Build history of the part. All positions in model axes, mm. Coordinates: 2 decimals unless noted, no trailing zeros. Write each loop counter-clockwise with the first axis right and the second up, starting at its lowest first coordinate (ties: lowest second). Pieces come first, ordered by that corner, then holes. Notation, with made-up numbers: (72, 12.25) -> (95, 12.25) arc R30 cw to (95, 39.25) -> close; hole circle Ø8 at (6.25, -29). An arc over 180 degrees is marked (long way). Write each question's results on one line, items separated by ' | '. Start each with the question number.
Q1. Drill centre lines: line 1 (Z direction, x = 3.25, y = -1.45); line 2 (Y direction, x = -0.5, z = 1.8); line 3 (X direction, y = 0.5, z = 1.8). Where is each one in solid material? Low to high.
Q2. Saw through at B-B on z = 0.75. Give the cut face in (x, y) (1 decimal), and give its area (3 significant figures).
Q3. Saw through at C-C on z = 1.45. Give the cut face in (x, y), and give its area (3 significant figures).
Q4. Saw through at A-A on x = -1. Give the cut face in (y, z) (1 decimal), and give its area (3 significant figures).
Q5. Saw through at D-D on y = -1.65. Give the cut face in (x, z).
from build123d import *

# Parameters (mm, degrees)
F0_W     = 9.906
F0_H     = 4.191
F1_DEPTH = 1.27
F3_DEPTH = 0.635
F4_R     = 0.3175
F5_DEPTH = 25.4


with BuildPart() as f1:
    # F0 (on Top) → F1 (new body)
    with BuildSketch(Plane.XY):
        Rectangle(F0_W, F0_H)
    extrude(amount=F1_DEPTH)

    # F2 (on face) → F3 (join)
    with BuildSketch(Plane.XY.offset(1.27)):
        with BuildLine():
            ThreePointArc((3.81, 0), (3.438026, 0.898026), (2.54, 1.27))
            Line((2.54, 1.27), (-2.54, 1.27))
            ThreePointArc((-2.54, 1.27), (-3.438026, 0.898026), (-3.81, 0))
            ThreePointArc((-3.81, 0), (-3.438026, -0.898026), (-2.54, -1.27))
            Line((-2.54, -1.27), (2.54, -1.27))
            ThreePointArc((2.54, -1.27), (3.438026, -0.898026), (3.81, 0))
        make_face()
    extrude(amount=F3_DEPTH)

    # F4 (on face) → F5 (cut)
    with BuildSketch(Plane.XY.offset(1.27)):
        with Locations((4.422641, 0)):
            Circle(F4_R)
        with Locations((-4.389373, 0)):
            Circle(F4_R)
    extrude(amount=-F5_DEPTH, mode=Mode.SUBTRACT)


solid = f1.part
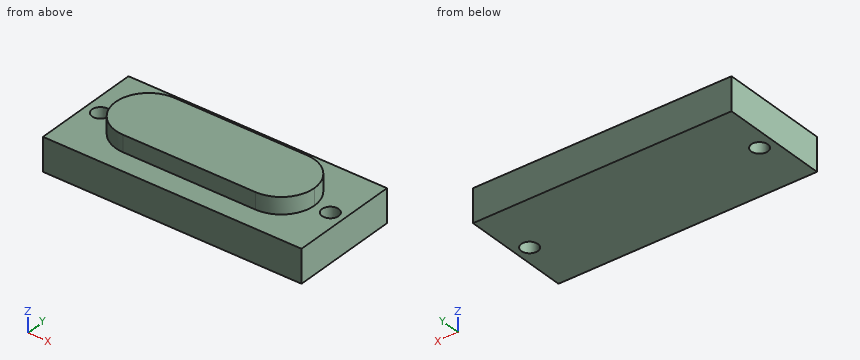
Returned:
1) line 1: z = 0 to 1.27 | line 2: y = -1.27 to 1.27 | line 3: x = -3.71 to 3.71
2) outline: (-5, -2.1) -> (5, -2.1) -> (5, 2.1) -> (-5, 2.1) -> close; hole circle Ø0.6 at (-4.4, 0); hole circle Ø0.6 at (4.4, 0) | area: 40.9 mm2
3) outline: (-3.81, 0) arc R1.27 ccw to (-2.54, -1.27) -> (2.54, -1.27) arc R1.27 ccw to (3.81, 0) arc R1.27 ccw to (2.54, 1.27) -> (-2.54, 1.27) arc R1.27 ccw to start | area: 18.0 mm2
4) outline: (-2.1, 0) -> (2.1, 0) -> (2.1, 1.3) -> (1.3, 1.3) -> (1.3, 1.9) -> (-1.3, 1.9) -> (-1.3, 1.3) -> (-2.1, 1.3) -> close | area: 6.94 mm2
5) outline: (-4.95, 0) -> (4.95, 0) -> (4.95, 1.27) -> (-4.95, 1.27) -> close
